Could you check a few things on this drawing? It's one solid part, dimensions in mm from its lowest x, y, z. Give positions to 0.01 mm unless a question says otherwise; leave off trailing zeros. Order: outer loops, then holes, each group sorted by start corner. A loop starts at its lowest first (then second) coordinate and runs counter-clockwise, first axis right, second up. Notation, with made-up numbers: M -10.5,-33 L 20.5,-33 A23 ccw 20.5,-20 Z; hole C 11.25,32 d2. An arc over 180 degrees is marked long. One line per item, written item: value. Start each with the question number.
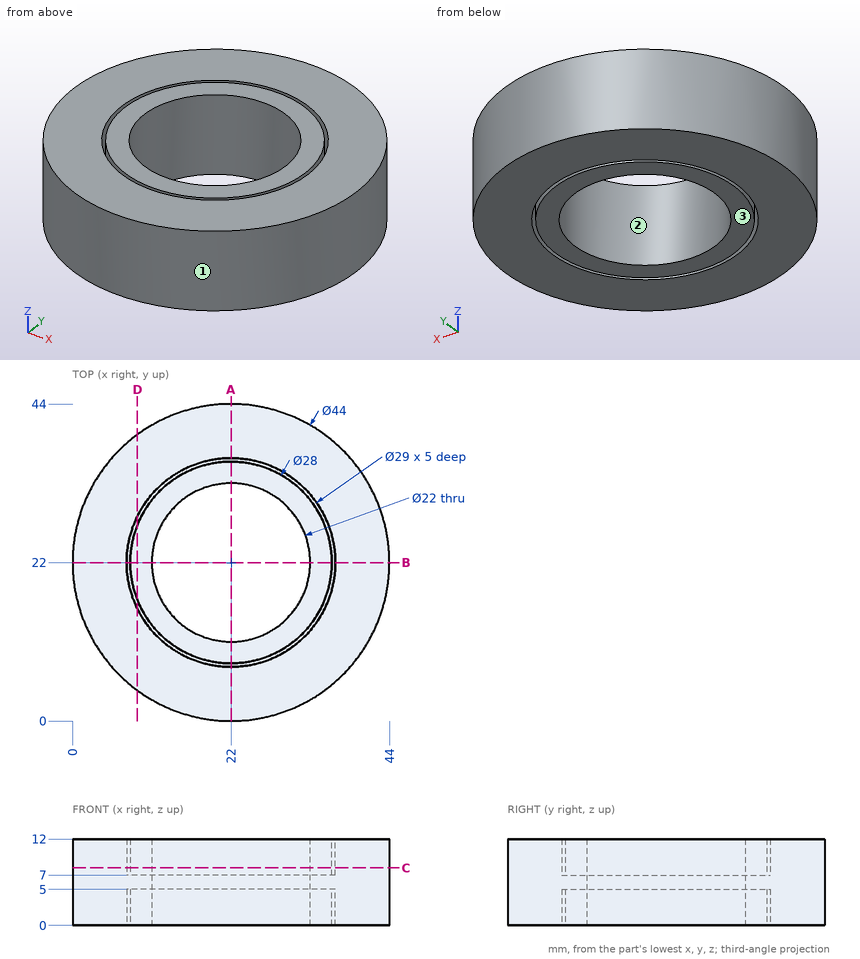
Item 1: I want a section at D-D on x = 9. Write out the boundary of the cut face in (y, z).
Item 2: Please list where these lines run through material, in increasing order: probe 1 along Y at (x, z) = (22, 9); probe 2 along X at (y, z) = (31, 1.75); probe 3 along X at (y, z) = (26, 3.5). Write a range as [from, to].
Item 3: We'd pull the mould along Y, two halves only. Please class the marked faces 1, 2 and 3: +Y half, -Y half, draft (parallel to the pull), parting line (faces both ways), or undercut.
Item 4: Will these pins go through, and if not, where does the flat tip stop? P1, Ø3, axis at x = 38, z = 4, coming from the +Y side; P2, Ø3, axis at y = 20.5, z = 8, coming from the -X side; P3, Ø2, axis at x = 25, z = 10.5, coming from the -Y side; P4, Ø1.5, axis at y = 29, z = 10.5, coming from the -X side.
Item 5: I want a section at C-C on z = 8. Write out the boundary of the cut face in (x, y), plus the area to 3 significant figures.
Item 6: I want a section at A-A on x = 22. Write out the boundary of the cut face in (y, z), plus the area to 3 significant figures.
Answer below:
1. outline: M 4.25,0 L 15.58,0 L 15.58,5 L 16.8,5 L 16.8,0 L 27.2,0 L 27.2,5 L 28.42,5 L 28.42,0 L 39.75,0 L 39.75,12 L 28.42,12 L 28.42,7 L 27.2,7 L 27.2,12 L 16.8,12 L 16.8,7 L 15.58,7 L 15.58,12 L 4.25,12 Z
2. probe 1: y = [0, 7.5], [8, 11], [33, 36], [36.5, 44]
2. probe 2: x = [1.93, 10.63], [11.28, 15.68], [28.32, 32.72], [33.37, 42.07]
2. probe 3: x = [0.37, 8.06], [8.58, 11.75], [32.25, 35.42], [35.94, 43.63]
3. face 1: parting line
3. face 2: undercut
3. face 3: draft
4. P1: stops at y = 38.55
4. P2: stops at x = 0
4. P3: stops at y = 0.09
4. P4: stops at x = 0.91
5. outline: C 22,22 d44; C 22,22 d28; hole C 22,22 d29; hole C 22,22 d22
5. area: 1,100 mm²
6. outline: M 0,0 L 7.5,0 L 7.5,5 L 8,5 L 8,0 L 11,0 L 11,12 L 8,12 L 8,7 L 7.5,7 L 7.5,12 L 0,12 Z; M 33,0 L 36,0 L 36,5 L 36.5,5 L 36.5,0 L 44,0 L 44,12 L 36.5,12 L 36.5,7 L 36,7 L 36,12 L 33,12 Z
6. area: 254 mm²
